from build123d import *

# Parameters (mm, degrees)
SKETCH1_W           = 76.2
SKETCH1_H           = 50.8
SKETCH1_W_2         = 63.5
SKETCH1_H_2         = 38.1
BOSS_EXTRUDE1_DEPTH = 114.3
SKETCH2_R           = 14.2875
CUT_EXTRUDE2_DEPTH  = 114.3
SKETCH3_W           = 63.5
SKETCH3_H           = 101.6
CUT_EXTRUDE3_DEPTH  = 7.62


with BuildPart() as part:
    # Sketch1 → Boss-Extrude1 (new body)
    with BuildSketch(Plane.XY):
        Rectangle(SKETCH1_W, SKETCH1_H)
        Rectangle(SKETCH1_W_2, SKETCH1_H_2, mode=Mode.SUBTRACT)
    extrude(amount=BOSS_EXTRUDE1_DEPTH)

    # Sketch2 → Cut-Extrude2 (cut)
    with BuildSketch(Plane(origin=(0, 25.4, 0), x_dir=(1, 0, 0), z_dir=(0, 1, 0))):
        with BuildLine():
            Line((38.1, -114.3), (38.1, -73.025))
            ThreePointArc((38.1, -73.025), (0, -98.425), (-38.1, -73.025))
            Line((-38.1, -73.025), (-38.1, -114.3))
            Line((-38.1, -114.3), (38.1, -114.3))
        make_face()
        with Locations((0, -57.15)):
            Circle(SKETCH2_R)
        with BuildLine():
            ThreePointArc((-38.1, -41.275), (0, -15.875), (38.1, -41.275))
            Line((38.1, -41.275), (38.1, 0))
            Line((38.1, 0), (-38.1, 0))
            Line((-38.1, 0), (-38.1, -41.275))
        make_face()
    extrude(amount=-CUT_EXTRUDE2_DEPTH, mode=Mode.SUBTRACT)

    # Sketch3 → Cut-Extrude3 (cut)
    with BuildSketch(Plane.XZ.offset(25.4)):
        with Locations((0, 57.15)):
            Rectangle(SKETCH3_W, SKETCH3_H)
    extrude(amount=-CUT_EXTRUDE3_DEPTH, mode=Mode.SUBTRACT)


solid = part.part
Geometry check sheet. Reference: the model listing, model coordinates, mm. A direction names the side the tool comes from. Round coordinates to 2 decimals unless told otherwise and drop trailing zeros. Loops run counter-clockwise (first coordinate to the right, second up) from the corner with the lowest first, then second, coordinate; pieces in that order, holes last.
Item 1: Mould release check, pull along Z, two halves, no side actions. Record for faces 3 (the cylindrical face through (-3.817, 20.815, 16.052)), 4 (the flat face through (-38.1, 0, 57)), 5 (the cylindrical face through (-3.097, 22.269, 71.098)): pulls with the +Z half, pulls with the -Z half, needs draft (parallel to the pull), parting line crosses it, or undercut.
Item 2: Thickness scan on line 1 (X direction, y = -17.5, z = 58.5); line 2 (X direction, y = 22.25, z = 57.15); line 3 (Z direction, x = 0, y = 23.75) (1 decimal). Record the ranges inside material, lowest first.
Item 3: Access from +Z, -Z, +X, -X, +Y, -Y to the whole of each face (thin tool, end or side, straight path). Record for faces 1 (the flat face through (-35, -25.4, 57)), 2 (the flat face through (31.75, -3, 57)).
Item 4: Cross-section at D-D on x = -22. Record the boundary of the cut face in (y, z).
Item 5: Cross-section at A-A on z = 57.15. Record the boundary of the cut face in (x, y).
Item 6: Cross-section at C-C on y = -6.5. Record the boundary of the cut face in (x, z) (3 decimals), then the cut area to 3 significant figures.
Item 7: Gauge pin test, flat ends, axial feed: pin 1 (19 mm diameter, centred on x = 1, z = 54, fed in from -Y); pin 2 (1 mm diameter, centred on y = -13, z = 82.5, fed in from -X); pin 3 (1 mm diameter, centred on y = 20, z = 74, fed in from +X); pin 4 (6 mm diameter, centred on x = 14, z = 42, fed in from -Y). Record the tip position at first contact, or that the pin passes through.
Answer sheet:
1. face 3: pulls with the -Z half
1. face 4: needs draft
1. face 5: undercut
2. line 1: x = -38.1 to -31.75, 31.75 to 38.1
2. line 2: x = -38.1 to -14.29, 14.29 to 38.1
2. line 3: z = 15.9 to 42.9, 71.4 to 98.4
3. face 1: +Z, -Z, +X, -X, -Y
3. face 2: +Z, -Z, -Y
4. outline: (19.05, 22.23) - (25.4, 22.23) - (25.4, 92.07) - (19.05, 92.07) - close
5. outline: (-38.1, -25.4) - (-31.75, -25.4) - (-31.75, 19.05) - (-14.29, 19.05) - (-14.29, 25.4) - (-38.1, 25.4) - close; (14.29, 19.05) - (31.75, 19.05) - (31.75, -25.4) - (38.1, -25.4) - (38.1, 25.4) - (14.29, 25.4) - close
6. outline: (-38.1, 41.275) arc R41.275 ccw to (-31.75, 30.776) - (-31.75, 83.524) arc R41.275 ccw to (-38.1, 73.025) - close; (31.75, 30.776) arc R41.275 ccw to (38.1, 41.275) - (38.1, 73.025) arc R41.275 ccw to (31.75, 83.524) - close
6. area: 552 mm2
7. pin 1: passes through
7. pin 2: stops at x = -32.96
7. pin 3: stops at x = 37.9
7. pin 4: stops at y = 19.05
